```python
from build123d import *

# Parameters (mm, degrees)
ESQUISSE2_R             = 1
BOSS_EXTRU_1_DEPTH      = 16.5
BOSS_EXTRU_1_DEPTH_BACK = 11
ESQUISSE3_R             = 2
BOSS_EXTRU_2_DEPTH      = 2
ESQUISSE4_OUTSIDE_W     = 12.008
ESQUISSE4_OUTSIDE_H     = 12.008
ENL_V_MAT_EXTRU_1_DEPTH = 30.5
CHANFREIN1_SIZE         = 0.5
ESQUISSE6_R             = 1
ENL_V_MAT_EXTRU_2_DEPTH = 4.5


with BuildPart() as part:
    # Esquisse2 → Boss.-Extru.1 (new body, two sides)
    with BuildSketch(Plane.XY) as boss_extru_1_sk:
        with Locations((0, 1.35)):
            Circle(ESQUISSE2_R)
    extrude(amount=BOSS_EXTRU_1_DEPTH)
    extrude(boss_extru_1_sk.sketch, amount=-BOSS_EXTRU_1_DEPTH_BACK)

    # Esquisse3 → Boss.-Extru.2 (add)
    with BuildSketch(Plane.XY.offset(16.5)):
        with Locations((0, 1.35)):
            Circle(ESQUISSE3_R)
    extrude(amount=BOSS_EXTRU_2_DEPTH)

    # Esquisse4 outside → Enlèv. mat.-Extru.1 (cut, through all)
    with BuildSketch(Plane.XY.offset(18.5)):
        with Locations((0, 1.35)):
            Rectangle(ESQUISSE4_OUTSIDE_W, ESQUISSE4_OUTSIDE_H)
        with BuildLine():
            Line((-1.3, 2.869868415), (-1.3, 0.05))
            Line((-1.3, 0.05), (1.3, 0.05))
            Line((1.3, 0.05), (1.3, 2.869868415))
            ThreePointArc((1.3, 2.869868415), (0, 3.35), (-1.3, 2.869868415))
        make_face(mode=Mode.SUBTRACT)
    extrude(amount=-ENL_V_MAT_EXTRU_1_DEPTH, mode=Mode.SUBTRACT)

    # Chanfrein1
    chanfrein1_edges = [part.edges().sort_by_distance(p)[0] for p in [
        (0, 0.05, 18.5),
    ]]
    chamfer(chanfrein1_edges, length=CHANFREIN1_SIZE)

    # Esquisse6 → Enlèv. mat.-Extru.2 (cut)
    with BuildSketch(Plane(origin=(0, 0, -11), x_dir=(-1, 0, 0), z_dir=(0, 0, -1))):
        with Locations((0, 1.35)):
            Circle(ESQUISSE6_R)
    extrude(amount=-ENL_V_MAT_EXTRU_2_DEPTH, mode=Mode.SUBTRACT)


solid = part.part
```
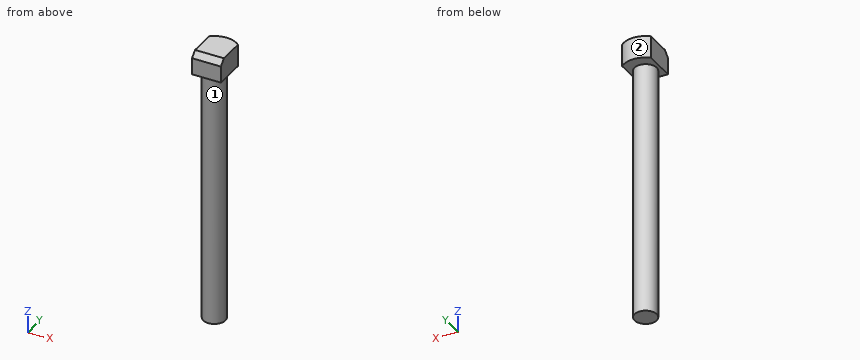
Design review of the part built by this model. Coordinates are the model's own, in mm. Face numbers are marked on the shaded views. A direction names the side the tool comes from. Coordinates: 2 decimals unless noted, no trailing zeros. Loops run counter-clockwise (first coordinate to the right, second up) from the corner with the lowest first, then second, coordinate; pieces in that order, holes last. Notation, with made-up numbers: (-20, 4) - (35, 4) arc R25 ccw to (35, 21) - close; hole circle Ø7 at (-13, -19). An arc over 180 degrees is marked (long way). Use CSV: the item, a comma, the result in double quotes. Start each with the question number.
1) Tool access review of the marked faces 1 and 2: name each direction out of +Z, -Z, +X, -X, +Y, -Y from which nothing blocks a thin tool from reaching the whole face with its end or side.
2) Wall thickness on L1, parallel to Z at x = -0.15, y = 2.5; L2, parallel to X at y = 1.3, z = 2.25; L3, parallel to Y at x = 0.15, z = 15: over which ranges is each line inside the solid? List them lowest first. Write a range as from..to.
3) Consider section A-A on y = 1.35. Write out the cut boundary in (x, z).
4) Consider section C-C on z = -3.5. Write out the cut boundary in (x, y), then the cut area to 3 significant figures.
5) Consider section B-B on x = 0. Write out the cut boundary in (y, z), then the cut area to 3 significant figures.
Geometry says:
1,face 1,"-Z"
1,face 2,"+Z, -Z, +Y"
2,L1,"16.5..18.5"
2,L2,"-1..1"
2,L3,"0.36..2.34"
3,outline,"(-1.3, 16.5) - (-1, 16.5) - (-1, -6.5) - (1, -6.5) - (1, 16.5) - (1.3, 16.5) - (1.3, 18.5) - (-1.3, 18.5) - close"
4,outline,"circle Ø2 at (0, 1.35)"
4,area,"3.14 mm^2"
5,outline,"(0.05, 16.5) - (0.35, 16.5) - (0.35, -6.5) - (2.35, -6.5) - (2.35, 16.5) - (3.35, 16.5) - (3.35, 18.5) - (0.55, 18.5) - (0.05, 18) - close"
5,area,"52.5 mm^2"
